The model under review builds one solid part; all positions refer to its coordinate system, in mm. A direction names the side the tool comes from. Give positions to 0.01 mm unless a question says otherwise; leave off trailing zeros. Order: outer loops, then holes, each group sorted by start corner. A loop starts at its lowest first (then second) coordinate and runs counter-clockwise, first axis right, second up. Notation, with made-up numbers: (31, -31.5) -> (58, -31.5) arc R5 cw to (58, -26.5) -> close; hole circle Ø9 at (-38, 34.5). An arc over 180 degrees is marked (long way). Use one line per item in the form item = value.
```python
from build123d import *

# Parameters (mm, degrees)
SKETCH_1_W      = 67.8
SKETCH_1_H      = 53
SKETCH_1_R      = 1.6
EXTRUDE_1_DEPTH = 1.2
SKETCH_2_W      = 25.4
SKETCH_2_H      = 2.54
SKETCH_2_W_2    = 20.32
SKETCH_2_W_3    = 15.24
SKETCH_2_W_4    = 2.54
SKETCH_2_H_2    = 12.7
EXTRUDE_2_DEPTH = 8
SKETCH_3_W      = 7.6
SKETCH_3_H      = 15
SKETCH_3_W_2    = 10
SKETCH_3_H_2    = 7.6
EXTRUDE_3_DEPTH = 9
CHAMFER_1_SIZE  = 2


with BuildPart() as part:
    # 草图1 → 凸台-拉伸1 (new body)
    with BuildSketch(Plane(origin=(0, 0, 0), x_dir=(1, 0, 0), z_dir=(0, 1, 0))):
        with Locations((33.9, 26.5)):
            Rectangle(SKETCH_1_W, SKETCH_1_H)
        with Locations(Location((64.8, 35, 0), (0, 0, 270))):
            Circle(SKETCH_1_R, mode=Mode.SUBTRACT)
        with Locations(Location((64.8, 7, 0), (0, 0, 270))):
            Circle(SKETCH_1_R, mode=Mode.SUBTRACT)
        with Locations(Location((14.4, 50.4, 0), (0, 0, 270))):
            Circle(SKETCH_1_R, mode=Mode.SUBTRACT)
    extrude(amount=EXTRUDE_1_DEPTH)

    # 草图2 → 凸台-拉伸2 (add)
    with BuildSketch(Plane(origin=(0, 1.2, 0), x_dir=(1, 0, 0), z_dir=(0, 1, 0))):
        with Locations((28.9, 50.41)):
            Rectangle(SKETCH_2_W, SKETCH_2_H)
        with Locations((53.03, 50.41)):
            Rectangle(SKETCH_2_W_2, SKETCH_2_H)
        with Locations((33.72, 2.54)):
            Rectangle(SKETCH_2_W_2, SKETCH_2_H)
        with Locations((54.06, 2.54)):
            Rectangle(SKETCH_2_W_3, SKETCH_2_H)
        with Locations((58.93, 37.35)):
            Rectangle(SKETCH_2_W_4, SKETCH_2_H_2)
    extrude(amount=EXTRUDE_2_DEPTH)

    # 草图3 → 凸台-拉伸3 (add)
    with BuildSketch(Plane(origin=(0, 1.2, 0), x_dir=(1, 0, 0), z_dir=(0, 1, 0))):
        with Locations((3.8, 23.16)):
            Rectangle(SKETCH_3_W, SKETCH_3_H)
        with Locations((17.42, 3.8)):
            Rectangle(SKETCH_3_W_2, SKETCH_3_H_2)
    extrude(amount=EXTRUDE_3_DEPTH)

    # 倒角1
    chamfer_1_edges = [part.edges().sort_by_distance(p)[0] for p in [
        (17.42, 10.2, -7.6),
        (7.6, 10.2, -23.16),
    ]]
    chamfer(chamfer_1_edges, length=CHAMFER_1_SIZE)


solid = part.part
```
1. Add section C-C on y = 7. Give the boundary of the cut face in (x, z), then the cut area to 3 significant figures.
Values:
outline = (0, -30.66) -> (7.6, -30.66) -> (7.6, -15.66) -> (0, -15.66) -> close; (12.42, -7.6) -> (22.42, -7.6) -> (22.42, 0) -> (12.42, 0) -> close; (16.2, -51.68) -> (41.6, -51.68) -> (41.6, -49.14) -> (16.2, -49.14) -> close; (23.56, -3.81) -> (43.88, -3.81) -> (43.88, -1.27) -> (23.56, -1.27) -> close; (42.87, -51.68) -> (63.19, -51.68) -> (63.19, -49.14) -> (42.87, -49.14) -> close; (46.44, -3.81) -> (61.68, -3.81) -> (61.68, -1.27) -> (46.44, -1.27) -> close; (57.66, -43.7) -> (60.2, -43.7) -> (60.2, -31) -> (57.66, -31) -> close
area = 429 mm^2
2. The part is to be moulded in two halves that separate along X. For faces 1 (the face through (63.19, 5, -50)), 2 (the face through (34, 9.2, -3)), 3 (the face through (41.6, 5, -50)), say which applies: +X half, -X half, draft (parallel to the pull), parting line (faces both ways), or undercut.
Values:
face_1 = +X half
face_2 = draft
face_3 = undercut
3. Add section B-B on z = -35. Give the boundary of the cut face in (x, y), then the cut area to 3 significant figures.
Values:
outline = (0, 0) -> (63.2, 0) -> (63.2, 1.2) -> (60.2, 1.2) -> (60.2, 9.2) -> (57.66, 9.2) -> (57.66, 1.2) -> (0, 1.2) -> close; (66.4, 0) -> (67.8, 0) -> (67.8, 1.2) -> (66.4, 1.2) -> close
area = 97.8 mm^2
4. Tool access review of faces 4 (the face through (22.42, 6, -4)), 5 (the face through (53, 5, -51.68)), 6 (the face through (61.68, 5, -3)): name each direction out of +Z, -Z, +X, -X, +Y, -Y from which nothing blocks a thin tool from reaching the whole face with its end or side.
Values:
face_4 = +Z, +Y
face_5 = -Z, +X, -X, +Y
face_6 = +Z, +X, +Y
5. Add section D-D on x = 64.8. Give the boundary of the cut face in (y, z).
Values:
outline = (0, -53) -> (1.2, -53) -> (1.2, -36.6) -> (0, -36.6) -> close; (0, -33.4) -> (1.2, -33.4) -> (1.2, -8.6) -> (0, -8.6) -> close; (0, -5.4) -> (1.2, -5.4) -> (1.2, 0) -> (0, 0) -> close
6. For L1, parallel to Z at x = 64.8, y = 0.9; L2, parallel to X at y = 0.4, z = -7; L3, parallel to Z at x = 57, y = 3, list the stretches that pass through material, from the lowest coordinate up.
Values:
L1 = -53 to -36.6, -33.4 to -8.6, -5.4 to 0
L2 = 0 to 63.2, 66.4 to 67.8
L3 = -51.68 to -49.14, -3.81 to -1.27
7. Add section A-A on x = 14.4. Give the boundary of the cut face in (y, z).
Values:
outline = (0, -53) -> (1.2, -53) -> (1.2, -52) -> (0, -52) -> close; (0, -48.8) -> (1.2, -48.8) -> (1.2, -7.6) -> (8.2, -7.6) -> (10.2, -5.6) -> (10.2, 0) -> (0, 0) -> close
8. For pin 1 Ø10 at (x, z) = (25, -23.5) entering from +Y; pin 2 Ø2 at (y, z) = (5.5, -51) entering from +X; pin 3 Ø2.5 at (x, z) = (14.4, -50.4) entering from -Y; pin 4 Ø2 at (y, z) = (6, -24) entering from +X, all flat-tipped, find the tip position at first contact; note any pin that passes through.
Values:
pin_1 = 1.2
pin_2 = 63.19
pin_3 = through
pin_4 = 7.6
